Here's how the part is built. I have some questions about the finished solid (model axes, mm). A direction names the side the tool comes from. Coordinates: 2 decimals unless noted, no trailing zeros. Order: outer loops, then holes, each group sorted by start corner. A loop starts at its lowest first (then second) coordinate and runs counter-clockwise, first axis right, second up. Notation, with made-up numbers: M -29.75,13 L -23.75,13 A9 cw -23.75,23 Z; hole C -9.5,-37 d8. An arc over 180 degrees is marked long. Answer as CSV lines item,"result". Start each with the question number.
```python
from build123d import *

# Parameters (mm, degrees)
BOSS_EXTRUDE1_DEPTH      = 20
BOSS_EXTRUDE1_DEPTH_BACK = 20
SKETCH1_W                = 35
SKETCH1_H                = 65.2
CUT_EXTRUDE3_REACH       = 92.614
SKETCH7_R                = 1.55
SKETCH7_R_2              = 2.9
CUT_EXTRUDE4_DEPTH       = 10
BOSS_EXTRUDE2_DEPTH      = 40


with BuildPart() as part:
    # Sketch1 → Boss-Extrude1 (new, two sides: drawn at the far end of the back side and taken through both)
    with BuildSketch(Plane.XY.offset(-BOSS_EXTRUDE1_DEPTH_BACK)):
        with Locations((6.633557164, -45.043181818)):
            Rectangle(SKETCH1_W, SKETCH1_H)
    extrude(amount=BOSS_EXTRUDE1_DEPTH + BOSS_EXTRUDE1_DEPTH_BACK)

    # Sketch5 → Cut-Extrude3 (cut, up to next)
    with BuildSketch(Plane.XY.offset(20), mode=Mode.PRIVATE) as cut_extrude3_sk1:
        with BuildLine():
            Line((-4.866442836, -31.243181818), (-4.866442836, -35.243181818))
            ThreePointArc((-4.866442836, -35.243181818), (-4.573549617, -35.950288599), (-3.866442836, -36.243181818))
            Line((-3.866442836, -36.243181818), (17.133557164, -36.243181818))
            ThreePointArc((17.133557164, -36.243181818), (17.840663945, -35.950288599), (18.133557164, -35.243181818))
            Line((18.133557164, -35.243181818), (18.133557164, -31.243181818))
            ThreePointArc((18.133557164, -31.243181818), (17.840663945, -30.536075037), (17.133557164, -30.243181818))
            Line((17.133557164, -30.243181818), (-3.866442836, -30.243181818))
            ThreePointArc((-3.866442836, -30.243181818), (-4.573549617, -30.536075037), (-4.866442836, -31.243181818))
        make_face()
    cut_extrude3_tool1 = extrude(cut_extrude3_sk1.sketch, amount=-CUT_EXTRUDE3_REACH, mode=Mode.PRIVATE) & part.part
    # Sketch5 → Cut-Extrude3 (cut, up to next)
    with BuildSketch(Plane.XY.offset(20), mode=Mode.PRIVATE) as cut_extrude3_sk2:
        with BuildLine():
            Line((-4.866442836, -43.043181818), (-4.866442836, -47.043181818))
            ThreePointArc((-4.866442836, -47.043181818), (-4.573549617, -47.750288599), (-3.866442836, -48.043181818))
            Line((-3.866442836, -48.043181818), (17.133557164, -48.043181818))
            ThreePointArc((17.133557164, -48.043181818), (17.840663945, -47.750288599), (18.133557164, -47.043181818))
            Line((18.133557164, -47.043181818), (18.133557164, -43.043181818))
            ThreePointArc((18.133557164, -43.043181818), (17.840663945, -42.336075037), (17.133557164, -42.043181818))
            Line((17.133557164, -42.043181818), (-3.866442836, -42.043181818))
            ThreePointArc((-3.866442836, -42.043181818), (-4.573549617, -42.336075037), (-4.866442836, -43.043181818))
        make_face()
    cut_extrude3_tool2 = extrude(cut_extrude3_sk2.sketch, amount=-CUT_EXTRUDE3_REACH, mode=Mode.PRIVATE) & part.part
    # Sketch5 → Cut-Extrude3 (cut, up to next)
    with BuildSketch(Plane.XY.offset(20), mode=Mode.PRIVATE) as cut_extrude3_sk3:
        with BuildLine():
            Line((-3.866442836, -18.443181818), (17.133557164, -18.443181818))
            ThreePointArc((17.133557164, -18.443181818), (17.840663945, -18.736075037), (18.133557164, -19.443181818))
            Line((18.133557164, -19.443181818), (18.133557164, -23.443181818))
            ThreePointArc((18.133557164, -23.443181818), (17.840663945, -24.150288599), (17.133557164, -24.443181818))
            Line((17.133557164, -24.443181818), (-3.866442836, -24.443181818))
            ThreePointArc((-3.866442836, -24.443181818), (-4.573549617, -24.150288599), (-4.866442836, -23.443181818))
            Line((-4.866442836, -23.443181818), (-4.866442836, -19.443181818))
            ThreePointArc((-4.866442836, -19.443181818), (-4.573549617, -18.736075037), (-3.866442836, -18.443181818))
        make_face()
    cut_extrude3_tool3 = extrude(cut_extrude3_sk3.sketch, amount=-CUT_EXTRUDE3_REACH, mode=Mode.PRIVATE) & part.part
    # Sketch5 → Cut-Extrude3 (cut, up to next)
    with BuildSketch(Plane.XY.offset(20), mode=Mode.PRIVATE) as cut_extrude3_sk4:
        with BuildLine():
            Line((-4.866442836, -54.843181818), (-4.866442836, -58.843181818))
            ThreePointArc((-4.866442836, -58.843181818), (-4.573549617, -59.550288599), (-3.866442836, -59.843181818))
            Line((-3.866442836, -59.843181818), (17.133557164, -59.843181818))
            ThreePointArc((17.133557164, -59.843181818), (17.840663945, -59.550288599), (18.133557164, -58.843181818))
            Line((18.133557164, -58.843181818), (18.133557164, -54.843181818))
            ThreePointArc((18.133557164, -54.843181818), (17.840663945, -54.136075037), (17.133557164, -53.843181818))
            Line((17.133557164, -53.843181818), (-3.866442836, -53.843181818))
            ThreePointArc((-3.866442836, -53.843181818), (-4.573549617, -54.136075037), (-4.866442836, -54.843181818))
        make_face()
    cut_extrude3_tool4 = extrude(cut_extrude3_sk4.sketch, amount=-CUT_EXTRUDE3_REACH, mode=Mode.PRIVATE) & part.part
    # Sketch5 → Cut-Extrude3 (cut, up to next)
    with BuildSketch(Plane.XY.offset(20), mode=Mode.PRIVATE) as cut_extrude3_sk5:
        with BuildLine():
            Line((-4.866442836, -66.643181818), (-4.866442836, -70.643181818))
            ThreePointArc((-4.866442836, -70.643181818), (-4.573549617, -71.350288599), (-3.866442836, -71.643181818))
            Line((-3.866442836, -71.643181818), (17.133557164, -71.643181818))
            ThreePointArc((17.133557164, -71.643181818), (17.840663945, -71.350288599), (18.133557164, -70.643181818))
            Line((18.133557164, -70.643181818), (18.133557164, -66.643181818))
            ThreePointArc((18.133557164, -66.643181818), (17.840663945, -65.936075037), (17.133557164, -65.643181818))
            Line((17.133557164, -65.643181818), (-3.866442836, -65.643181818))
            ThreePointArc((-3.866442836, -65.643181818), (-4.573549617, -65.936075037), (-4.866442836, -66.643181818))
        make_face()
    cut_extrude3_tool5 = extrude(cut_extrude3_sk5.sketch, amount=-CUT_EXTRUDE3_REACH, mode=Mode.PRIVATE) & part.part
    add(cut_extrude3_tool1.solids().sort_by_distance((6.633557, -33.243182, 20))[0], mode=Mode.SUBTRACT)
    add(cut_extrude3_tool2.solids().sort_by_distance((6.633557, -45.043182, 20))[0], mode=Mode.SUBTRACT)
    add(cut_extrude3_tool3.solids().sort_by_distance((6.633557, -21.443182, 20))[0], mode=Mode.SUBTRACT)
    add(cut_extrude3_tool4.solids().sort_by_distance((6.633557, -56.843182, 20))[0], mode=Mode.SUBTRACT)
    add(cut_extrude3_tool5.solids().sort_by_distance((6.633557, -68.643182, 20))[0], mode=Mode.SUBTRACT)

    # Sketch7 → Cut-Extrude4 (cut)
    with BuildSketch(Plane(origin=(0, -12.443181818, 0), x_dir=(1, 0, 0), z_dir=(0, 1, 0))):
        with Locations(Location((1.648454357, 4.985102807, 0), (0, 0, 270))):
            Circle(SKETCH7_R)
        with Locations(Location((6.633557164, 0, 0), (0, 0, 270))):
            Circle(SKETCH7_R_2)
        with Locations(Location((11.618659971, 4.985102807, 0), (0, 0, 270))):
            Circle(SKETCH7_R)
        with Locations(Location((11.618659971, -4.985102807, 0), (0, 0, 270))):
            Circle(SKETCH7_R)
        with Locations(Location((1.648454357, -4.985102807, 0), (0, 0, 270))):
            Circle(SKETCH7_R)
    cut_extrude4 = extrude(amount=-CUT_EXTRUDE4_DEPTH, mode=Mode.SUBTRACT)

    # Mirror5: Cut-Extrude4 across plane
    add(cut_extrude4.mirror(Plane.ZX.offset(-45.043181818)), mode=Mode.SUBTRACT)

    # Sketch9 → Boss-Extrude2 (add)
    with BuildSketch(Plane(origin=(0, 0, -20), x_dir=(-1, 0, 0), z_dir=(0, 0, -1))):
        with BuildLine():
            Line((-24.133557164, -24.855210359), (-24.133557164, -12.443181818))
            Line((-24.133557164, -12.443181818), (-26.165618229, -12.443181818))
            ThreePointArc((-26.165618229, -12.443181818), (-27.91889587, -13.480883782), (-27.852793861, -15.517164307))
            Line((-27.852793861, -15.517164307), (-26.01050337, -18.411315428))
            ThreePointArc((-26.01050337, -18.411315428), (-24.612345302, -21.499368105), (-24.133557164, -24.855210359))
        make_face()
        with BuildLine():
            Line((-24.133557164, -77.643181818), (-24.133557164, -65.231153277))
            ThreePointArc((-24.133557164, -65.231153277), (-24.612345302, -68.586995532), (-26.01050337, -71.675048209))
            Line((-26.01050337, -71.675048209), (-27.852793861, -74.56919933))
            ThreePointArc((-27.852793861, -74.56919933), (-27.91889587, -76.605479855), (-26.165618229, -77.643181818))
            Line((-26.165618229, -77.643181818), (-24.133557164, -77.643181818))
        make_face()
        with BuildLine():
            Line((10.866442836, -65.231153277), (10.866442836, -77.643181818))
            Line((10.866442836, -77.643181818), (12.898503901, -77.643181818))
            ThreePointArc((12.898503901, -77.643181818), (14.651781542, -76.605479855), (14.585679533, -74.56919933))
            Line((14.585679533, -74.56919933), (12.743389042, -71.675048209))
            ThreePointArc((12.743389042, -71.675048209), (11.345230974, -68.586995532), (10.866442836, -65.231153277))
        make_face()
        with BuildLine():
            Line((10.866442836, -12.443181818), (10.866442836, -24.855210359))
            ThreePointArc((10.866442836, -24.855210359), (11.345230974, -21.499368105), (12.743389042, -18.411315428))
            Line((12.743389042, -18.411315428), (14.585679533, -15.517164307))
            ThreePointArc((14.585679533, -15.517164307), (14.651781542, -13.480883782), (12.898503901, -12.443181818))
            Line((12.898503901, -12.443181818), (10.866442836, -12.443181818))
        make_face()
    extrude(amount=-BOSS_EXTRUDE2_DEPTH)


solid = part.part
```
1) Suppose I cut it at A-A on x = 16. Please give me the cut outline in (y, z), plus the area to 3 significant figures.
2) Will these pins go through, and if not, where does the flat tip stop? pin 1 Ø3 at (y, z) = (-44, -2.5) entering from +X; pin 2 Ø1 at (y, z) = (-61.5, 4) entering from -X; pin 3 Ø2.5 at (x, z) = (11.62, 4.99) entering from +Y.
3) Which directions (+Z, -Z, +X, -X, +Y, -Y) give clear straight access to the entire face, cutting with the end or side of a thin tool? Please do faces 4 (the face through (2.114, -74.685, -3.507)), 5 (the face through (7, -42.043, 0)), 6 (the face through (26.919, -73.102, -0.28)).
4) Suppose I cut it at B-B on z = 5.5. Give the number of separate pieces and of enclosed holes in the cut face, plus the area to 3 significant figures.
5) If we mould it in two halves opening along X, with no side actions, what happens to faces 1 (the face through (11, -77.643, 0)), 2 (the face through (-11.359, -68.633, -0.28)), 3 (the face through (12.926, -74.685, -4.152))? For each: released by +X, released by -X, zero draft, split by the parting line, or undercut.
6) Suppose I cut it at C-C on y = -16.5. Please give me the cut outline in (x, z), plus the area to 3 significant figures.
7) I need wall thicknesses on line 1 (Y direction, x = 6.5, z = -17); line 2 (Y direction, x = 7, z = 2); line 3 (X direction, y = -16.5, z = 5.5). Which ranges of each line are inside material? Lowest first, please. Write a range as [from, to].
Output:
1,outline,"M -77.64,-20 L -71.64,-20 L -71.64,20 L -77.64,20 Z; M -65.64,-20 L -59.84,-20 L -59.84,20 L -65.64,20 Z; M -53.84,-20 L -48.04,-20 L -48.04,20 L -53.84,20 Z; M -42.04,-20 L -36.24,-20 L -36.24,20 L -42.04,20 Z; M -30.24,-20 L -24.44,-20 L -24.44,20 L -30.24,20 Z; M -18.44,-20 L -12.44,-20 L -12.44,20 L -18.44,20 Z"
1,area,"1,410 mm²"
2,pin 1,"x = 24.13"
2,pin 2,"x = -10.87"
2,pin 3,"y = -24.44"
3,face 4,"-Y"
3,face 5,"+Z, -Z"
3,face 6,"+Z, -Z, +X"
4,separate pieces,"3"
4,enclosed holes,"3"
4,area,"1,620 mm²"
5,face 1,"zero draft"
5,face 2,"released by -X"
5,face 3,"undercut"
6,outline,"M -13.96,-20 L 27.23,-20 L 27.23,20 L -13.96,20 Z; hole C 1.65,-4.99 d3.1; hole C 1.65,4.99 d3.1; hole C 6.63,0 d5.8; hole C 11.62,-4.99 d3.1; hole C 11.62,4.99 d3.1"
6,area,"1,590 mm²"
7,line 1,"[-77.64, -71.64], [-65.64, -59.84], [-53.84, -48.04], [-42.04, -36.24], [-30.24, -24.44], [-18.44, -12.44]"
7,line 2,"[-65.64, -59.84], [-53.84, -48.04], [-42.04, -36.24], [-30.24, -24.44]"
7,line 3,"[-13.96, 0.19], [3.11, 10.16], [13.08, 27.23]"
